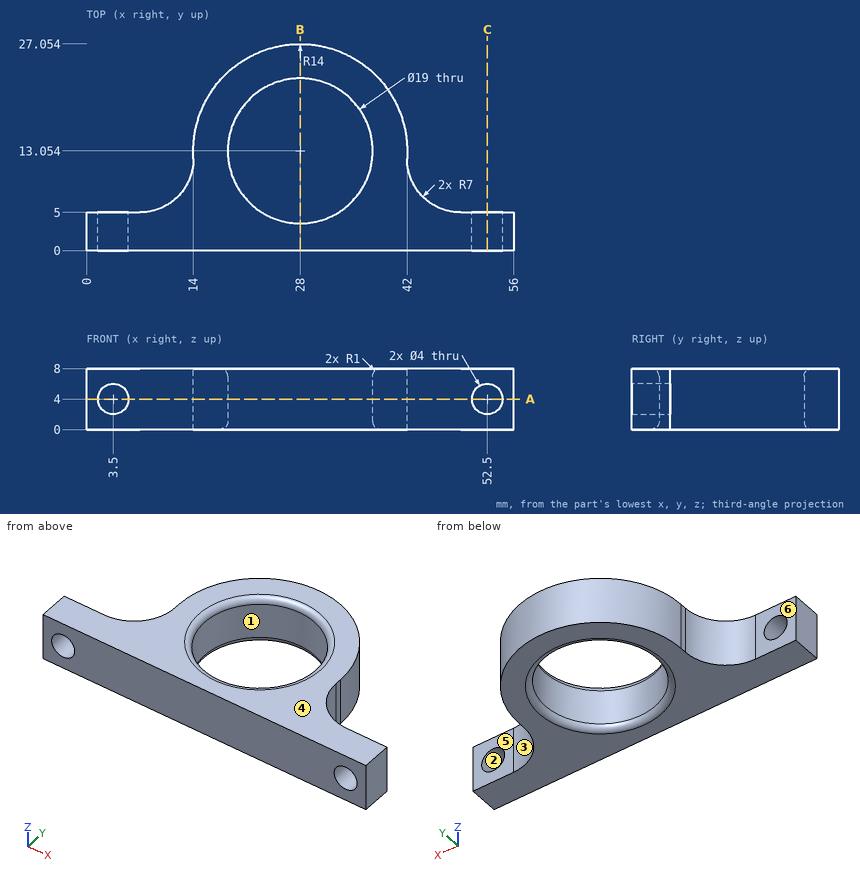
Part print with two shaded views. Sizes in mm from the minimum x, y, z corner. A direction names the side the tool comes from. Coordinates: 2 decimals unless noted, no trailing zeros. Order: outer loops, then holes, each group sorted by start corner. A loop starts at its lowest first (then second) coordinate and runs counter-clockwise, first axis right, second up. Notation, with made-up numbers: M 36.5,-15.5 L 43.5,-15.5 A29 ccw 43.5,15.5 Z; hole C -30,40.5 d5. An arc over 180 degrees is marked long. Use a Markdown table: item, result.
(1) Flat gauge pins, fed straight in: pin 1 (2.5 mm diameter, centred on x = 3.5, z = 4, fed in from +Y); pin 2 (1 mm diameter, centred on y = 13.5, z = 2.5, fed in from -X); pin 3 (2 mm diameter, centred on x = 31.5, z = 6.5, fed in from -Y); pin 4 (2 mm diameter, centred on x = 47, z = 3.5, fed in from +Y) (1 decimal). Where does each tip first touch, or does it go through?
A:
| item | result |
|---|---|
| pin 1 | passes through |
| pin 2 | stops at x = 14 |
| pin 3 | stops at y = 0 |
| pin 4 | stops at y = 5.7 |
(2) Probe L1, parallel to X at y = 1.35, z = 4; L2, parallel to Y at x = 28, z = 2.6; L3, parallel to Y at x = 6.5, z = 2.75. List the from-to ranges inside material, lowest first.
A:
| item | result |
|---|---|
| L1 | x = 0 to 1.5, 5.5 to 50.5, 54.5 to 56 |
| L2 | y = 0 to 3.55, 22.55 to 27.05 |
| L3 | y = 0 to 5 |
(3) Pull direction Y, two halves, no side cores. Call the marked faces 1, 2 and 3: released by +Y, released by -Y, zero draft, split by the parting line, or undercut.
A:
| item | result |
|---|---|
| face 1 | undercut |
| face 2 | zero draft |
| face 3 | released by +Y |
(4) Cut at C-C on x = 52.5. Write the cut outline in (y, z), then the cut area to 3 significant figures.
A:
| item | result |
|---|---|
| outline | M 0,0 L 5,0 L 5,2 L 0,2 Z; M 0,6 L 5,6 L 5,8 L 0,8 Z |
| area | 20.0 mm^2 |
(5) Tool access for the marked faces 4, 5 and 6: list every direction of +Z, -Z, +X, -X, +Y, -Y with a clear straight run to the whole face (end or side of a thin tool).
A:
| item | result |
|---|---|
| face 4 | +Z, +X, -X, +Y, -Y |
| face 5 | +Z, -Z, +X, +Y |
| face 6 | +Z, -Z, -X, +Y |
(6) Cut at B-B on x = 28. Write the cut outline in (y, z).
A:
| item | result |
|---|---|
| outline | M 0,0 L 2.55,0 A1 ccw 3.55,1 L 3.55,7 A1 ccw 2.55,8 L 0,8 Z; M 22.55,1 A1 ccw 23.55,0 L 27.05,0 L 27.05,8 L 23.55,8 A1 ccw 22.55,7 Z |
(7) Cut at A-A on z = 4. Write the cut outline in (x, y), then the cut area to 3 significant figures.
A:
| item | result |
|---|---|
| outline | M 0,0 L 1.5,0 L 1.5,5 L 0,5 Z; M 5.5,0 L 50.5,0 L 50.5,5 L 49,5 A7 cw 42,12 L 42,13.05 A14 ccw 14,13.05 L 14,12 A7 cw 7,5 L 5.5,5 Z; M 54.5,0 L 56,0 L 56,5 L 54.5,5 Z; hole C 28,13.05 d19 |
| area | 511 mm^2 |
